from build123d import *

# Parameters (mm, degrees)
F0_W      = 47.7
F0_H      = 9.6
F0_R      = 2.4
F1_DEPTH  = 9.5
F2_DEPTH  = 2.2
F3_W      = 44.25676
F3_H      = 6.6
F3_R      = 1.55
F3_R_2    = 2.072202
F1_FACE_W = 47.7
F1_FACE_H = 9.6
F4_DEPTH  = 2
F5_W      = 44.538753
F5_H      = 6.894205
F6_DEPTH  = 10.15
F7_R      = 1.55
F8_DEPTH  = 10.15


with BuildPart() as f1:
    # F0 (on Top) → F1 (new body)
    with BuildSketch(Plane.XY):
        Rectangle(F0_W, F0_H)
        with Locations((-20.25, 0)):
            Circle(F0_R, mode=Mode.SUBTRACT)
        with Locations((-12.65, 0)):
            Circle(F0_R, mode=Mode.SUBTRACT)
        with Locations((-5.05, 0)):
            Circle(F0_R, mode=Mode.SUBTRACT)
        with Locations((5.05, 0)):
            Circle(F0_R, mode=Mode.SUBTRACT)
        with Locations((12.65, 0)):
            Circle(F0_R, mode=Mode.SUBTRACT)
        with Locations((20.25, 0)):
            Circle(F0_R, mode=Mode.SUBTRACT)
        with Locations((-20.25, 0)):
            Circle(F0_R)
        with Locations((-12.65, 0)):
            Circle(F0_R)
        with Locations((-5.05, 0)):
            Circle(F0_R)
        with Locations((5.05, 0)):
            Circle(F0_R)
        with Locations((12.65, 0)):
            Circle(F0_R)
        with Locations((20.25, 0)):
            Circle(F0_R)
    extrude(amount=F1_DEPTH)

    # F0 (on Top) → F2 (join)
    with BuildSketch(Plane.XY):
        with Locations((-20.25, 0)):
            Circle(F0_R)
        with Locations((-12.65, 0)):
            Circle(F0_R)
        with Locations((-5.05, 0)):
            Circle(F0_R)
        with Locations((5.05, 0)):
            Circle(F0_R)
        with Locations((12.65, 0)):
            Circle(F0_R)
        with Locations((20.25, 0)):
            Circle(F0_R)
    extrude(amount=-F2_DEPTH)

    # F3 (on Top) + F1_face (on face) → F4 (join)
    with BuildSketch(Plane.XY):
        Rectangle(F3_W, F3_H)
        with Locations((-19.1, 0)):
            Circle(F3_R, mode=Mode.SUBTRACT)
        with Locations((-12.5, 0)):
            Circle(F3_R, mode=Mode.SUBTRACT)
        Circle(F3_R_2, mode=Mode.SUBTRACT)
        with Locations((12.524975, 0)):
            Circle(F3_R, mode=Mode.SUBTRACT)
        with Locations((19.124975, 0)):
            Circle(F3_R, mode=Mode.SUBTRACT)
    with BuildSketch(Plane.XY.offset(9.5)):
        Rectangle(F1_FACE_W, F1_FACE_H)
    extrude(amount=F4_DEPTH)

    # F5 (on face) → F6 (cut)
    with BuildSketch(Plane.XY.offset(11.5)):
        with Locations((0.013958, 0.144912)):
            Rectangle(F5_W, F5_H)
    extrude(amount=-F6_DEPTH, mode=Mode.SUBTRACT)

    # F7 (on face) → F8 (join)
    with BuildSketch(Plane.XY.offset(1.35)):
        with Locations((-17.37838, 0)):
            Circle(F7_R)
        with Locations((-9.27838, 0)):
            Circle(F7_R)
        Circle(F7_R)
        with Locations((8.69896, 0)):
            Circle(F7_R)
        with Locations((16.79896, 0)):
            Circle(F7_R)
    extrude(amount=F8_DEPTH)


solid = f1.part
Input: part model. Units: mm. Frame: model coordinates. A direction names the side the tool comes from. Give positions to 0.01 mm unless a question says otherwise; leave off trailing zeros. Write each loop counter-clockwise with the first axis right and the second up, starting at its lowest first coordinate (ties: lowest second). Pieces come first, ordered by that corner, then holes. Notation, with made-up numbers: M 49.25,4 L 102.25,4 A30 cw 102.25,31 Z; hole C 45,-0.5 d5. An arc over 180 degrees is marked long. Write item = value, one per line. Start each with the question number.
1) Reachability of faces 4 (the cylindrical face through (7.34, 0.72, -1.08)), 5 (the flat face through (9, 0, 11.5)), 6 (the flat face through (0, -3.302, 6)) from +Z, -Z, +X, -X, +Y, -Y: full face, straight path, thin tool, end or side. Return the list, or none.
2) Material intervals for line 1 along Y through (x, z) = (14, 4); line 2 along X through (y, z) = (-1.5, -0.5); line 3 along X through (y, z) = (-2, 6.5), sorted ascending. Write a range as [from, to].
3) Cut plane B-B on x = 0. Return the cut outline in (y, z), then the cut area to 3 significant figures.
4) Cut plane A-A on z = 10. Return the cut outline in (x, y), then the cut area to 3 significant figures.
5) Draft query along Y for faces 1 (the cylindrical face through (0.715, -1.375, 6.354)), 2 (the flat face through (0, 0, 0)), 3 (the cylindrical face through (-17.96, 0.72, -1.08)). Return one class per face: +Y half, -Y half, draft (parallel to the pull), parting line (faces both ways), or undercut.
6) Cut plane C-C on y = 4. Return the cut outline in (x, z).
7) Cut plane D-D on x = -20.25. Return the cut outline in (y, z).
Solved:
q1.face_4 = -Z
q1.face_5 = +Z, +X, -X, +Y, -Y
q1.face_6 = +Z
q2.line_1 = [-4.8, -3.3], [3.59, 4.8]
q2.line_2 = [-22.12, -18.38], [-14.52, -10.78], [-6.92, -3.18], [3.18, 6.92], [10.78, 14.52], [18.38, 22.12]
q2.line_3 = [-23.85, -22.26], [22.28, 23.85]
q3.outline = M -4.8,0 L 4.8,0 L 4.8,11.5 L 3.59,11.5 L 3.59,1.35 L 1.55,1.35 L 1.55,11.5 L -1.55,11.5 L -1.55,1.35 L -3.3,1.35 L -3.3,11.5 L -4.8,11.5 Z
q3.area = 71.9 mm2
q4.outline = M -23.85,-4.8 L 23.85,-4.8 L 23.85,4.8 L -23.85,4.8 Z; C -17.38,0 d3.1; C -9.28,0 d3.1; C 0,0 d3.1; C 8.7,0 d3.1; C 16.8,0 d3.1; hole M -22.26,-3.3 L 22.28,-3.3 L 22.28,3.59 L -22.26,3.59 Z
q4.area = 189 mm2
q5.face_1 = undercut
q5.face_2 = draft
q5.face_3 = parting line
q6.outline = M -23.85,0 L 23.85,0 L 23.85,11.5 L -23.85,11.5 Z
q7.outline = M -4.8,0 L -2.4,0 L -2.4,-2.2 L 2.4,-2.2 L 2.4,0 L 4.8,0 L 4.8,11.5 L 3.59,11.5 L 3.59,1.35 L -3.3,1.35 L -3.3,11.5 L -4.8,11.5 Z
